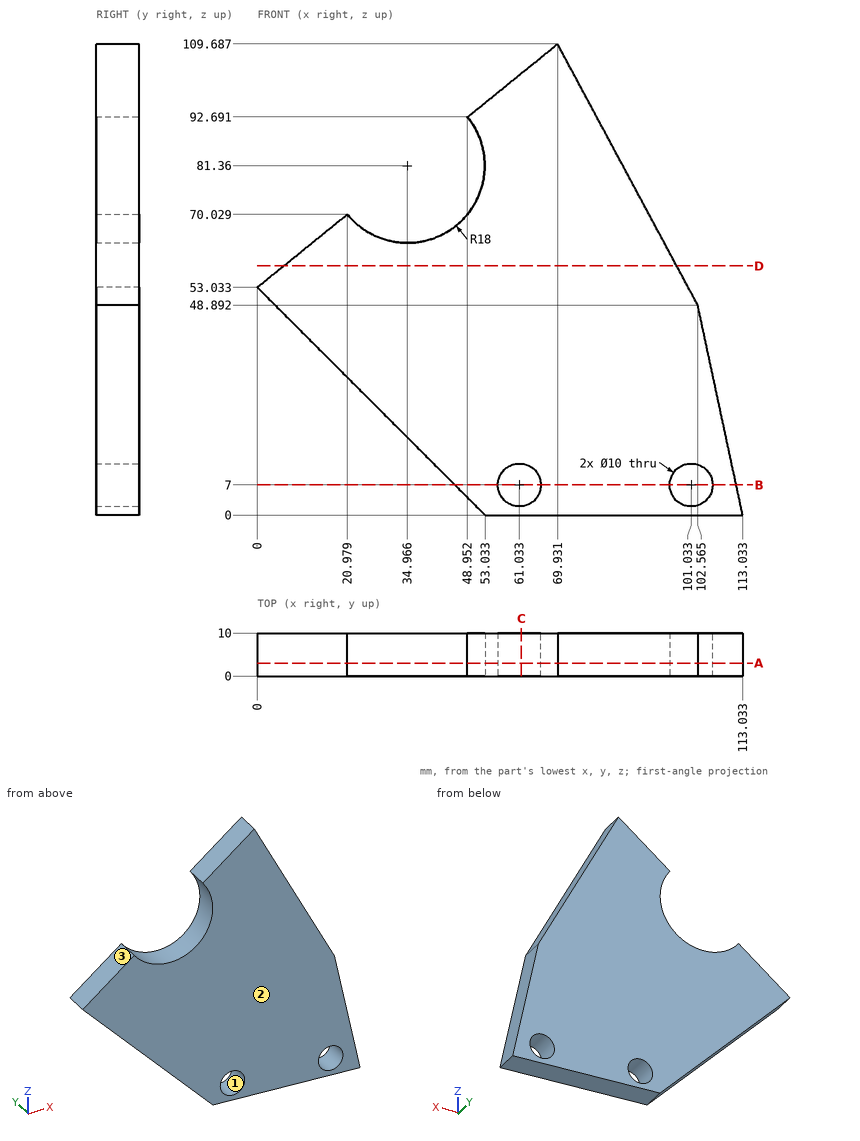
Geometry check sheet. Reference: drawing and pictorial views, mm from the part's lowest x, y, z. Round coordinates to 2 decimals unless told otherwise and drop trailing zeros. Order: outer loops, then holes, each group sorted by start corner. A loop starts at its lowest first (then second) coordinate and runs counter-clockwise, first axis right, second up. Notation, with made-up numbers: (-17.75, -37.75) - (37.25, -37.75) arc R31 ccw to (37.25, -5.75) - close; hole circle Ø5 at (40, -26.75). An arc over 180 degrees is marked (long way). Use a Markdown table: item, result. Add a question column.
1) Mould release check, pull along X, two halves, no side actions. Record for the marked faces 1, 2 and 3: released by +X, released by -X, zero draft, split by the parting line, or undercut.
2) Section check D-D (z = 58). Record the cut outline in (x, y) (1 decimal).
3) Section check C-C (x = 61.5). Record the cut outline in (y, z).
4) Thickness scan on line 1 along Z through (x, y) = (98.5, 1.5) (1 decimal); line 2 along X through (y, z) = (9.5, 5.5) (1 decimal); line 3 along Z through (x, y) = (99, 2.5) (1 decimal). Record the ranges inside material, lowest first.
5) Section check A-A (y = 3). Record the cut outline in (x, z) (1 decimal), then the cut area to 3 significant figures.
6) Section check B-B (z = 7). Record the cut outline in (x, y) (1 decimal), then the cut area to 3 significant figures.
7) Gauge pin test, flat ends, axial feed: P1, Ø4, axis at x = 30.5, y = 2, coming from the +Z side; P2, Ø1.5, axis at y = 5, z = 72.5, coming from the -X side (1 decimal); P3, Ø4, axis at x = 41, y = 8.5, coming from the +Z side; P4, Ø11.5, axis at x = 61.033, z = 7, coming from the +Y side. Record the tip position at first contact, or that the pin passes through.
Established:
| question | item | result |
|---|---|---|
| 1 | face 1 | undercut |
| 1 | face 2 | zero draft |
| 1 | face 3 | released by -X |
| 2 | outline | (6.1, 0) - (97.7, 0) - (97.7, 10) - (6.1, 10) - close |
| 3 | outline | (0, 0) - (10, 0) - (10, 2.02) - (0, 2.02) - close; (0, 11.98) - (10, 11.98) - (10, 102.86) - (0, 102.86) - close |
| 4 | line 1 | 0 to 2.7, 11.3 to 56.5 |
| 4 | line 2 | 47.5 to 56.3, 65.8 to 96.3, 105.8 to 111.9 |
| 4 | line 3 | 0 to 2.4, 11.6 to 55.5 |
| 5 | outline | (0, 53) - (53, 0) - (113, 0) - (102.6, 48.9) - (69.9, 109.7) - (49, 92.7) arc R18 cw to (21, 70) - close; hole circle Ø10 at (61, 7); hole circle Ø10 at (101, 7) |
| 5 | area | 6,460 mm2 |
| 6 | outline | (46, 0) - (56, 0) - (56, 10) - (46, 10) - close; (66, 0) - (96, 0) - (96, 10) - (66, 10) - close; (106, 0) - (111.5, 0) - (111.5, 10) - (106, 10) - close |
| 6 | area | 455 mm2 |
| 7 | P1 | z = 64.56 |
| 7 | P2 | x = 50.2 |
| 7 | P3 | z = 65.25 |
| 7 | P4 | y = 10 |
